Geometry: final body of the model. Coordinates: model frame, mm. Face numbers are marked on the shaded views. A direction names the side the tool comes from. Give positions to 0.01 mm unless a question says otherwise; leave off trailing zeros. Order: outer loops, then holes, each group sorted by start corner. A loop starts at its lowest first (then second) coordinate and runs counter-clockwise, first axis right, second up. Notation, with made-up numbers: (57.25, 33.5) -> (84.25, 33.5) arc R19 ccw to (84.25, 61.5) -> close; hole circle Ø7 at (17.25, -24). An arc over 180 degrees is marked (long way). One line per question, with ' | ' between items. Start each with the question number.
(1) Section A-A (x = -17). Return loops of the section in (y, z), then the cut area to 3 significant figures.
(2) Set-up query: the marked faces 1, 2, 3, 4 and 5. Return all of +Z, -Z, +X, -X, +Y, -Y with unobstructed straight access to the full face (end or side cutting, diameter ignored); none if empty.
(3) First-contact query: pin 1 Ø1 at (x, z) = (12, -21.5) entering from -Y; pin 2 Ø3 at (x, z) = (-0.5, -20.5) entering from -Y; pin 3 Ø3.5 at (y, z) = (22.5, -19) entering from -X; pin 4 Ø11 at (y, z) = (17.5, -19) entering from -X. Flat tips, straight axial feed; report the tip coordinate or a pass-through.
(4) Mould query, pull axis Z, two halves, no side actions, for the marked faces 6, 7 and 8. Classes: +Z half, -Z half, draft (parallel to the pull), parting line (faces both ways), or undercut.
(5) Section B-B (y = 15). Return loops of the section in (x, z), then the cut area to 3 significant figures.
(6) Ray query, L1, parallel to Y at x = -17, z = 0; L2, parallel to Z at x = 2.5, y = 18.25; L3, parallel to X at y = 5.75, z = -20.5. Return the intervals inside material, ascending.
(7) Section D-D (z = -6). Return loops of the section in (x, y).
(8) Section C-C (y = 20). Return loops of the section in (x, z), then the cut area to 3 significant figures.
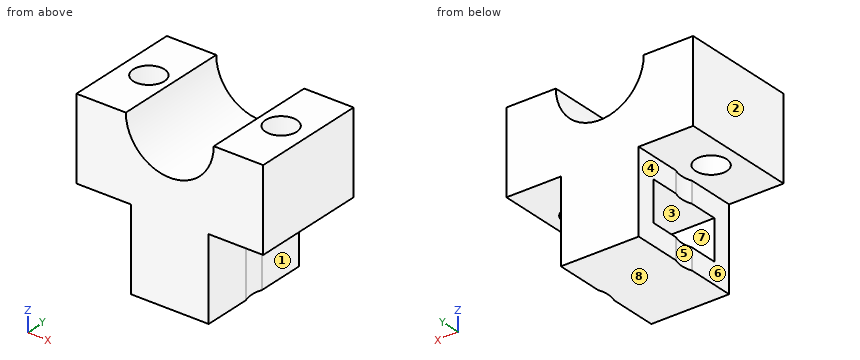
```python
from build123d import *

# Parameters (mm, degrees)
SKETCH_1_W          = 48
SKETCH_1_H          = 20
EXTRUDE_1_DEPTH     = 30
SKETCH_2_W          = 14
SKETCH_2_H          = 30
CUT_EXTRUDE_1_DEPTH = 7
SKETCH_7_W          = 22
SKETCH_7_H          = 30
EXTRUDE_2_DEPTH     = 48
SKETCH_8_W          = 21
SKETCH_8_H          = 30
CUT_EXTRUDE_2_DEPTH = 14
SKETCH_9_W          = 21
SKETCH_9_H          = 30
CUT_EXTRUDE_3_DEPTH = 14
SKETCH_11_W         = 10.2
SKETCH_11_H         = 20.2
CUT_EXTRUDE_4_DEPTH = 56.497747702
SKETCH_13_R         = 4
CUT_EXTRUDE_5_DEPTH = 44.783558558
SKETCH_14_R         = 4
CUT_EXTRUDE_6_DEPTH = 44.783558558
FILLET_1_R          = 7
SKETCH1_W           = 10.2
SKETCH1_H           = 20.2
BOSS_EXTRUDE1_DEPTH = 4
SKETCH_20_R         = 7.5
CUT_EXTRUDE_8_DEPTH = 44.783558558
SKETCH2_R           = 11.3
CUT_EXTRUDE1_DEPTH  = 51


with BuildPart() as part:
    # Эскиз1 → Бобышка-Вытянуть1 (new body)
    with BuildSketch(Plane(origin=(0, 0, 0), x_dir=(1, 0, 0), z_dir=(0, 1, 0))):
        Rectangle(SKETCH_1_W, SKETCH_1_H)
    extrude(amount=EXTRUDE_1_DEPTH)

    # Эскиз2 → Вырез-Вытянуть1 (cut)
    with BuildSketch(Plane.XY.offset(10)):
        with Locations((0, 15)):
            Rectangle(SKETCH_2_W, SKETCH_2_H)
    extrude(amount=-CUT_EXTRUDE_1_DEPTH, mode=Mode.SUBTRACT)

    # Эскиз7 → Бобышка-Вытянуть2 (add)
    with BuildSketch(Plane(origin=(24, 0, 0), x_dir=(0, 0, -1), z_dir=(1, 0, 0))):
        with Locations((21, 15)):
            Rectangle(SKETCH_7_W, SKETCH_7_H)
    extrude(amount=-EXTRUDE_2_DEPTH)

    # Эскиз8 → Вырез-Вытянуть2 (cut)
    with BuildSketch(Plane(origin=(24, 0, 0), x_dir=(0, 0, -1), z_dir=(1, 0, 0))):
        with Locations((21.5, 15)):
            Rectangle(SKETCH_8_W, SKETCH_8_H)
    extrude(amount=-CUT_EXTRUDE_2_DEPTH, mode=Mode.SUBTRACT)

    # Эскиз9 → Вырез-Вытянуть3 (cut)
    with BuildSketch(Plane.ZY.offset(24)):
        with Locations((-21.5, 15)):
            Rectangle(SKETCH_9_W, SKETCH_9_H)
    extrude(amount=-CUT_EXTRUDE_3_DEPTH, mode=Mode.SUBTRACT)

    # Эскиз11 → Вырез-Вытянуть4 (cut, through all)
    with BuildSketch(Plane.ZY.offset(10)):
        with Locations((-21.5, 15)):
            Rectangle(SKETCH_11_W, SKETCH_11_H)
    extrude(amount=-CUT_EXTRUDE_4_DEPTH, mode=Mode.SUBTRACT)

    # Эскиз13 → Вырез-Вытянуть5 (cut, through all)
    with BuildSketch(Plane(origin=(0, 0, -11), x_dir=(-1, 0, 0), z_dir=(0, 0, -1))):
        with Locations((17, 15)):
            Circle(SKETCH_13_R)
    extrude(amount=-CUT_EXTRUDE_5_DEPTH, mode=Mode.SUBTRACT)

    # Эскиз14 → Вырез-Вытянуть6 (cut, through all)
    with BuildSketch(Plane(origin=(0, 0, -11), x_dir=(-1, 0, 0), z_dir=(0, 0, -1))):
        with Locations((-17, 15)):
            Circle(SKETCH_14_R)
    extrude(amount=-CUT_EXTRUDE_6_DEPTH, mode=Mode.SUBTRACT)

    # Скругление1
    fillet_1_edges = [part.edges().sort_by_distance(p)[0] for p in [
        (-7, 15, 3),
        (7, 15, 3),
    ]]
    fillet(fillet_1_edges, radius=FILLET_1_R - 0.0001)  # a hair under: the kernel refuses the full size

    # Sketch1 → Boss-Extrude1 (add)
    with BuildSketch(Plane(origin=(10, 0, 0), x_dir=(0, 0, -1), z_dir=(1, 0, 0))):
        with Locations((21.5, 15)):
            Rectangle(SKETCH1_W, SKETCH1_H)
    extrude(amount=-BOSS_EXTRUDE1_DEPTH)

    # Эскиз20 → Вырез-Вытянуть8 (cut, through all)
    with BuildSketch(Plane(origin=(0, 0, -11), x_dir=(-1, 0, 0), z_dir=(0, 0, -1))):
        with Locations((-17, 15)):
            Circle(SKETCH_20_R)
        with Locations((17, 15)):
            Circle(SKETCH_20_R)
    extrude(amount=CUT_EXTRUDE_8_DEPTH, mode=Mode.SUBTRACT)

    # Sketch2 → Cut-Extrude1 (cut, through all)
    with BuildSketch(Plane(origin=(0, 30, 0), x_dir=(1, 0, 0), z_dir=(0, 1, 0))):
        with Locations((0, -10)):
            Circle(SKETCH2_R)
    extrude(amount=-CUT_EXTRUDE1_DEPTH, mode=Mode.SUBTRACT)


solid = part.part
```
Response:
1) outline: (0, -11) -> (11, -11) -> (11, 10) -> (0, 10) -> close; (19, -11) -> (30, -11) -> (30, 10) -> (19, 10) -> close | area: 462 mm^2
2) face 1: -Z, +X, +Y, -Y | face 2: +Z, -Z, -X, +Y, -Y | face 3: -X | face 4: -Z, -X, +Y, -Y | face 5: -Z, -X
3) pin 1: passes through | pin 2: stops at y = 0 | pin 3: stops at x = 6 | pin 4: stops at x = -10
4) face 6: draft | face 7: undercut | face 8: -Z half
5) outline: (-24, -11) -> (-21, -11) -> (-21, 10) -> (-24, 10) -> close; (-13, -11) -> (-9.5, -11) -> (-9.5, -16.4) -> (6, -16.4) -> (6, -26.6) -> (-9.5, -26.6) -> (-9.5, -32) -> (9.5, -32) -> (9.5, -11) -> (13, -11) -> (13, 10) -> (11.3, 10) arc R11.3 cw to (-11.3, 10) -> (-13, 10) -> close; (21, -11) -> (24, -11) -> (24, 10) -> (21, 10) -> close | area: 712 mm^2
6) L1: y = 0 to 11, 19 to 30 | L2: z = -32 to -26.6, -16.4 to -1.02 | L3: x = 6 to 10
7) outline: (-24, 0) -> (24, 0) -> (24, 30) -> (-24, 30) -> close; hole circle Ø8 at (-17, 15); hole circle Ø8 at (17, 15)
8) outline: (-24, -11) -> (-10, -11) -> (-10, -16.4) -> (6, -16.4) -> (6, -26.6) -> (-10, -26.6) -> (-10, -32) -> (10, -32) -> (10, -11) -> (24, -11) -> (24, 10) -> (11.3, 10) arc R11.3 cw to (-11.3, 10) -> (-24, 10) -> close | area: 1,060 mm^2
